```python
from build123d import *

# Parameters (mm, degrees)
F0_R     = 10.5
F0_R_2   = 1
F1_DEPTH = 15
F3_DEPTH = 13


# Not quite as in the source:
# - a feature names something its author has since deleted; it is built from what else it names


with BuildPart() as f1:
    # F0 (on Top) → F1 (new body)
    with BuildSketch(Plane.XY):
        with BuildLine():
            ThreePointArc((8.456539156, -32.2861623243), (7.9514162152, -32.0818291381), (7.456539156, -31.853798586))
            Line((7.456539156, -31.853798586), (4.5923320267, -38.8217959812))
            ThreePointArc((4.5923320267, -38.8217959812), (5.0983332026, -39.0569597997), (5.5923320267, -39.3163906642))
            Line((5.5923320267, -39.3163906642), (8.456539156, -32.2861623243))
        make_face()
        with BuildLine():
            ThreePointArc((5.5923320267, -39.3163906642), (5.0983332026, -39.0569597997), (4.5923320267, -38.8217959812))
            ThreePointArc((4.5923320267, -38.8217959812), (-0.2431846168, -37.8676348758), (-5.0340313362, -39.025405292))
            ThreePointArc((-5.0340313362, -39.025405292), (-5.4788213716, -39.2540536763), (-5.9132495676, -39.5018245418))
            ThreePointArc((-5.9132495676, -39.5018245418), (-9.7372709203, -43.2466031538), (-11.4521142662, -48.3166937306))
            ThreePointArc((-11.4521142662, -48.3166937306), (-11.4854214601, -48.7861903947), (-11.4994890326, -49.2566567486))
            ThreePointArc((-11.4994890326, -49.2566567486), (-8.2643935059, -57.3619252212), (-0.2699309272, -60.8618949578))
            ThreePointArc((-0.2699309272, -60.8618949578), (0.0361142384, -60.8650066318), (0.3421338242, -60.8599728394))
            ThreePointArc((0.3421338242, -60.8599728394), (8.2138697006, -57.4138113488), (11.4994866281, -49.473724691))
            ThreePointArc((11.4994866281, -49.473724691), (11.4998716563, -49.4193946208), (11.5, -49.365063338))
            ThreePointArc((11.5, -49.365063338), (11.4920706677, -48.9380835162), (11.4682936055, -48.5116925056))
            ThreePointArc((11.4682936055, -48.5116925056), (9.6904401721, -43.1726995509), (5.5923320267, -39.3163906642))
        make_face()
        with Locations((0, -49.365063338)):
            Circle(F0_R, mode=Mode.SUBTRACT)
        with BuildLine():
            Line((-5.0340313362, -39.025405292), (-7.8453759782, -31.8516950865))
            ThreePointArc((-7.8453759782, -31.8516950865), (-8.3405737258, -32.0678131455), (-8.8453759782, -32.2604332653))
            Line((-8.8453759782, -32.2604332653), (-5.9132495676, -39.5018245418))
            ThreePointArc((-5.9132495676, -39.5018245418), (-5.4788213716, -39.2540536763), (-5.0340313362, -39.025405292))
        make_face()
        with BuildLine():
            ThreePointArc((-11.4994890326, -49.2566567486), (-11.4854214601, -48.7861903947), (-11.4521142662, -48.3166937306))
            Line((-11.4521142662, -48.3166937306), (-14.3962585951, -47.6607659595))
            ThreePointArc((-14.3962585951, -47.6607659595), (-14.5881725993, -48.0436522978), (-14.7942107467, -48.4191269505))
            Line((-14.7942107467, -48.4191269505), (-11.4994890326, -49.2566567486))
        make_face()
        with BuildLine():
            Line((0.3421338242, -64.957754564), (0.3421338242, -60.8599728394))
            ThreePointArc((0.3421338242, -60.8599728394), (0.0361142384, -60.8650066318), (-0.2699309272, -60.8618949578))
            Line((-0.2699309272, -60.8618949578), (-0.2699309272, -64.9580295419))
            ThreePointArc((-0.2699309272, -64.9580295419), (0.0361017663, -64.9585994764), (0.3421338242, -64.957754564))
        make_face()
        with BuildLine():
            ThreePointArc((14.5406251326, -48.6339542886), (14.3126656094, -48.2217915649), (14.1017745949, -47.8006400066))
            Line((14.1017745949, -47.8006400066), (11.4682936055, -48.5116925056))
            ThreePointArc((11.4682936055, -48.5116925056), (11.4920706677, -48.9380835162), (11.5, -49.365063338))
            ThreePointArc((11.5, -49.365063338), (11.4998716563, -49.4193946208), (11.4994866281, -49.473724691))
            Line((11.4994866281, -49.473724691), (14.5406251326, -48.6339542886))
        make_face()
        with BuildLine():
            ThreePointArc((-18.6290237609, -32.9777593238), (-19.1442423903, -32.6707574729), (-19.6747657372, -32.391033768))
            ThreePointArc((-19.6747657372, -32.391033768), (-35.9088169714, -39.8355359758), (-25.2809881049, -54.1887337442))
            ThreePointArc((-25.2809881049, -54.1887337442), (-23.804958589, -54.1593636462), (-22.3448544462, -53.9411398473))
            ThreePointArc((-22.3448544462, -53.9411398473), (-17.9826996587, -51.9825521015), (-14.7942107467, -48.4191269505))
            ThreePointArc((-14.7942107467, -48.4191269505), (-14.5881725993, -48.0436522978), (-14.3962585951, -47.6607659595))
            ThreePointArc((-14.3962585951, -47.6607659595), (-13.5560532822, -45.2433801805), (-13.2712837616, -42.7000348848))
            ThreePointArc((-13.2712837616, -42.7000348848), (-14.6993924296, -37.1496290442), (-18.6290237609, -32.9777593238))
        make_face()
        with Locations((-24.7712837616, -42.7000348848)):
            Circle(F0_R, mode=Mode.SUBTRACT)
        with BuildLine():
            ThreePointArc((19.1164688634, -69.8349915238), (19.4845895022, -61.444857772), (23.9814303791, -54.3520248186))
            ThreePointArc((23.9814303791, -54.3520248186), (22.6698061738, -54.2185580929), (21.3820772546, -53.9358468382))
            ThreePointArc((21.3820772546, -53.9358468382), (18.3981233109, -58.1037903348), (16.5083411563, -62.8687098028))
            ThreePointArc((16.5083411563, -62.8687098028), (8.4897865212, -64.4127490141), (0.3421338242, -64.957754564))
            ThreePointArc((0.3421338242, -64.957754564), (0.0361017663, -64.9585994764), (-0.2699309272, -64.9580295419))
            ThreePointArc((-0.2699309272, -64.9580295419), (-8.785207594, -64.3721937184), (-17.154313878, -62.6955302663))
            ThreePointArc((-17.154313878, -62.6955302663), (-19.5673016908, -58.2102584784), (-22.3448544462, -53.9411398473))
            ThreePointArc((-22.3448544462, -53.9411398473), (-23.804958589, -54.1593636462), (-25.2809881049, -54.1887337442))
            ThreePointArc((-25.2809881049, -54.1887337442), (-20.5000187239, -61.334576051), (-19.5788875855, -69.8828067405))
            ThreePointArc((-19.5788875855, -69.8828067405), (-0.2273681462, -72.9674740069), (19.1164688634, -69.8349915238))
        make_face()
        with Locations((-15.5739570037, -67.6103085279)):
            Circle(F0_R_2, mode=Mode.SUBTRACT)
        with Locations((15.4391750693, -67.6299035549)):
            Circle(F0_R_2, mode=Mode.SUBTRACT)
        with BuildLine():
            ThreePointArc((-1.1916347077, -21.4227077758), (-1.1916502185, -21.4038200259), (-1.1916967507, -21.384932327))
            ThreePointArc((-1.1916967507, -21.384932327), (-18.3019531043, -11.3840660604), (-18.7497462956, -31.1976391816))
            ThreePointArc((-18.7497462956, -31.1976391816), (-18.319020566, -31.4517919016), (-17.8776520238, -31.6869770823))
            ThreePointArc((-17.8776520238, -31.6869770823), (-13.4202987359, -32.8995997215), (-8.8453759782, -32.2604332653))
            ThreePointArc((-8.8453759782, -32.2604332653), (-8.3405737258, -32.0678131455), (-7.8453759782, -31.8516950865))
            ThreePointArc((-7.8453759782, -31.8516950865), (-3.2683745706, -28.0145336524), (-1.2331773275, -22.3993113114))
            ThreePointArc((-1.2331773275, -22.3993113114), (-1.2020250565, -21.9114511274), (-1.1916347077, -21.4227077758))
        make_face()
        with Locations((-12.6916347077, -21.4227077758)):
            Circle(F0_R, mode=Mode.SUBTRACT)
        with BuildLine():
            ThreePointArc((-17.8776520238, -31.6869770823), (-18.319020566, -31.4517919016), (-18.7497462956, -31.1976391816))
            Line((-18.7497462956, -31.1976391816), (-19.6747657372, -32.391033768))
            ThreePointArc((-19.6747657372, -32.391033768), (-19.1442423903, -32.6707574729), (-18.6290237609, -32.9777593238))
            Line((-18.6290237609, -32.9777593238), (-17.8776520238, -31.6869770823))
        make_face()
        with BuildLine():
            ThreePointArc((1.0484752677, -22.3993113114), (1.0211177974, -21.8924785724), (1.0161513841, -21.384932327))
            Line((1.0161513841, -21.384932327), (-1.1916967507, -21.384932327))
            ThreePointArc((-1.1916967507, -21.384932327), (-1.1916502185, -21.4038200259), (-1.1916347077, -21.4227077758))
            ThreePointArc((-1.1916347077, -21.4227077758), (-1.2020250565, -21.9114511274), (-1.2331773275, -22.3993113114))
            Line((-1.2331773275, -22.3993113114), (1.0484752677, -22.3993113114))
        make_face()
        with BuildLine():
            ThreePointArc((19.2285761762, -30.8633233175), (22.7488768974, -26.7724999097), (24.0152835635, -21.5262090793))
            ThreePointArc((24.0152835635, -21.5262090793), (12.5859232723, -10.0264260365), (1.0161513841, -21.384932327))
            ThreePointArc((1.0161513841, -21.384932327), (1.0211177974, -21.8924785724), (1.0484752677, -22.3993113114))
            ThreePointArc((1.0484752677, -22.3993113114), (2.9958137546, -27.97831684), (7.456539156, -31.853798586))
            ThreePointArc((7.456539156, -31.853798586), (7.9514162152, -32.0818291381), (8.456539156, -32.2861623243))
            ThreePointArc((8.456539156, -32.2861623243), (13.3927953164, -32.9926807739), (18.1640607336, -31.5432603661))
            ThreePointArc((18.1640607336, -31.5432603661), (18.7056608481, -31.2179183751), (19.2285761762, -30.8633233175))
        make_face()
        with Locations((12.5152835635, -21.5262090793)):
            Circle(F0_R, mode=Mode.SUBTRACT)
        with BuildLine():
            Line((19.9216749616, -32.3085805793), (19.2285761762, -30.8633233175))
            ThreePointArc((19.2285761762, -30.8633233175), (18.7056608481, -31.2179183751), (18.1640607336, -31.5432603661))
            Line((18.1640607336, -31.5432603661), (18.8762154015, -32.8253023654))
            ThreePointArc((18.8762154015, -32.8253023654), (19.3923910412, -32.5536807799), (19.9216749616, -32.3085805793))
        make_face()
        with BuildLine():
            ThreePointArc((35.9878958911, -42.8631827235), (30.8021044444, -33.251691146), (19.9216749616, -32.3085805793))
            ThreePointArc((19.9216749616, -32.3085805793), (19.3923910412, -32.5536807799), (18.8762154015, -32.8253023654))
            ThreePointArc((18.8762154015, -32.8253023654), (13.5312723299, -39.3699893221), (14.1017745949, -47.8006400066))
            ThreePointArc((14.1017745949, -47.8006400066), (14.3126656094, -48.2217915649), (14.5406251326, -48.6339542886))
            ThreePointArc((14.5406251326, -48.6339542886), (17.4435150212, -51.9531056143), (21.3820772546, -53.9358468382))
            ThreePointArc((21.3820772546, -53.9358468382), (22.6698061738, -54.2185580929), (23.9814303791, -54.3520248186))
            ThreePointArc((23.9814303791, -54.3520248186), (32.4385451291, -51.1720440591), (35.9878958911, -42.8631827235))
        make_face()
        with Locations((24.4878958911, -42.8631827235)):
            Circle(F0_R, mode=Mode.SUBTRACT)
    extrude(amount=F1_DEPTH)

    # F2 (on face) → F3 (cut)
    with BuildSketch(Plane.XY.offset(15)):
        with BuildLine():
            Line((-25.4734057233, -63.6063340564), (-25.4734057233, -67.6063340564))
            ThreePointArc((-25.4734057233, -67.6063340564), (-0.2376476142, -73.3314436205), (24.9858820328, -67.5526964371))
            Line((24.9858820328, -67.5526964371), (24.9858820328, -63.5526964371))
            ThreePointArc((24.9858820328, -63.5526964371), (-0.2410172674, -66.1614613713), (-25.4734057233, -63.6063340564))
        make_face()
    extrude(amount=-F3_DEPTH, mode=Mode.SUBTRACT)


solid = f1.part
```
Source: CAD feature listing. Evaluate the final solid. Frame: model axes, mm. Round coordinates to 2 decimals unless told otherwise and drop trailing zeros. Order: outer loops, then holes, each group sorted by start corner. A loop starts at its lowest first (then second) coordinate and runs counter-clockwise, first axis right, second up. Notation, with made-up numbers: (47.25, -2.75) -> (100.25, -2.75) arc R21 ccw to (100.25, 17.25) -> close; hole circle Ø8 at (-29.75, 2). An arc over 180 degrees is marked (long way). One line per item, written item: value. Start each with the question number.
Q1. Draft query along Y for faces 1 (the cylindrical face through (-13.485, -32.895, 7.395)), 2 (the cylindrical face through (-0.14, -66.16, 8.59)), 3 (the cylindrical face through (14.44, -67.59, 0.99)). Return one class per face: pulls with the +Y half, pulls with the -Y half, needs draft (parallel to the pull), parting line crosses it, or undercut.
Q2. Section query B-B (y = -35). Return the cut outline in (x, z), plus the area to 3 significant figures.
Q3. Material intervals for probe 1 along X at (y, z) = (-59, 7); probe 2 along Y at (x, z) = (-19, 3.75); probe 3 along Y at (x, z) = (-3, 5.5), sorted ascending.
Q4. Section query C-C (z = 9.75). Give the number of separate pieces and of enclosed holes in the cut face, plus the area to 3 significant figures.
Q5. Section query A-A (y = -59). Return the cut outline in (x, z).
Q6. Pin query (flat end, axial travel): pin 1 (1 mm diameter, centred on x = 11, z = 8, fed in from +Y); pin 2 (1.2 mm diameter, centred on y = -64, z = 5.5, fed in from +X); pin 3 (0.7 mm diameter, centred on x = 0.5, z = 8.5, fed in from -Y); pin 4 (1.5 mm diameter, centred on x = 8, y = -47, fed in from -Z). Return the tip coordinate at first contact, or that it passes through.
Findings below:
1. face 1: undercut
1. face 2: pulls with the -Y half
1. face 3: undercut
2. outline: (-33.31, 0) -> (-31.91, 0) -> (-31.91, 15) -> (-33.31, 15) -> close; (-17.63, 0) -> (-16.23, 0) -> (-16.23, 15) -> (-17.63, 15) -> close; (-7.74, 0) -> (-6.61, 0) -> (-6.61, 15) -> (-7.74, 15) -> close; (6.16, 0) -> (7.35, 0) -> (7.35, 15) -> (6.16, 15) -> close; (16.1, 0) -> (17.53, 0) -> (17.53, 15) -> (16.1, 15) -> close; (31.45, 0) -> (32.88, 0) -> (32.88, 15) -> (31.45, 15) -> close
2. area: 120 mm²
3. probe 1: -21.54 to -19.11, -6.28 to -4.17, 4.17 to 6.28, 17.94 to 20.48
3. probe 2: -64.76 to -59.19, -52.65 to -51.47, -33.93 to -31.52, -31.04 to -29.82, -13.03 to -11.81
3. probe 3: -66.13 to -64.89, -60.47 to -59.43, -39.3 to -38.26, -27.61 to -25.46, -17.38 to -15.23
4. separate pieces: 1
4. enclosed holes: 10
4. area: 483 mm²
5. outline: (-21.54, 0) -> (-19.11, 0) -> (-19.11, 15) -> (-21.54, 15) -> close; (-6.28, 0) -> (-4.17, 0) -> (-4.17, 15) -> (-6.28, 15) -> close; (4.17, 0) -> (6.28, 0) -> (6.28, 15) -> (4.17, 15) -> close; (17.94, 0) -> (20.48, 0) -> (20.48, 15) -> (17.94, 15) -> close
6. pin 1: y = -10.07
6. pin 2: x = 19
6. pin 3: y = -66.16
6. pin 4: through
